The figure shows three views and two pictorial views of one solid part (mm, origin at its lowest corner). Answer the questions. A direction names the side the tool comes from. Give positions to 0.01 mm unless a question says otherwise; leave off trailing zeros. Order: outer loops, then holes, each group sorted by start corner. A loop starts at its lowest first (then second) coordinate and runs counter-clockwise, first axis right, second up. Notation, with made-up numbers: (48, -11) - (98, -11) arc R13 ccw to (98, 7) - close; hole circle Ø5 at (-35, 48.5). An arc over 180 degrees is marked (long way). Answer as CSV lines item,"result". Start each with the question number.
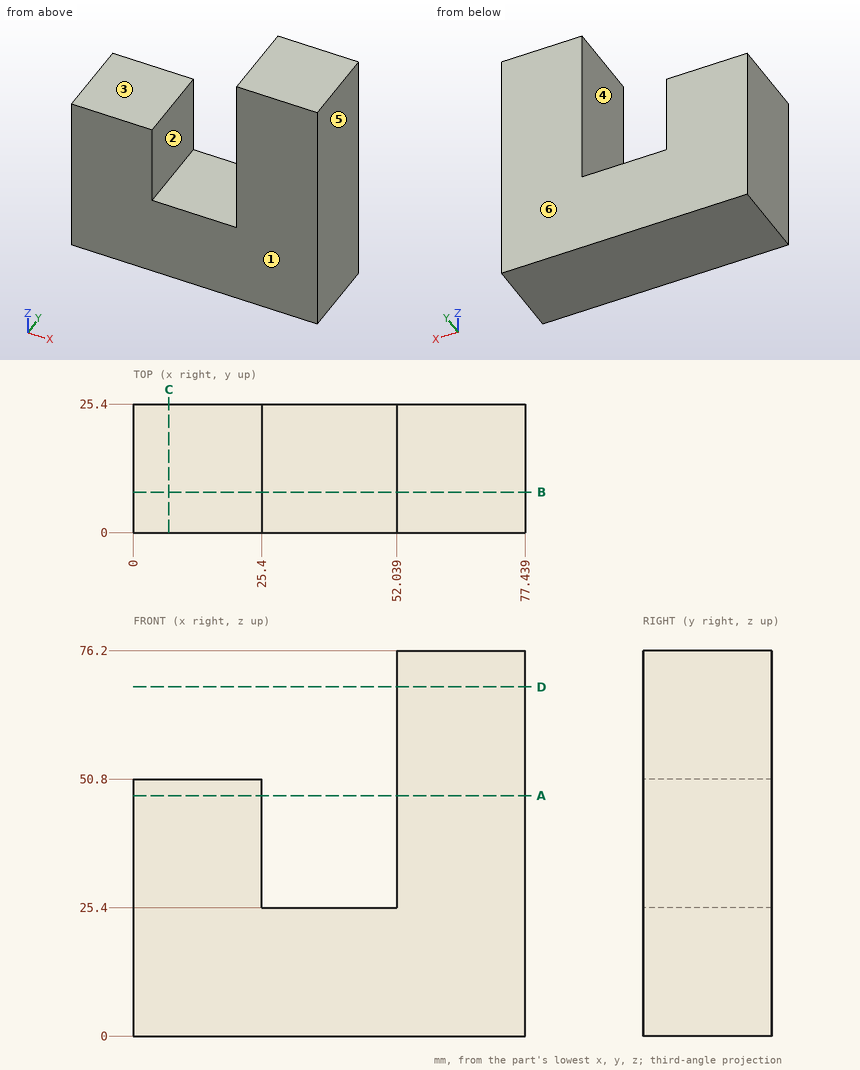
(1) Which of the six approach directions +Z, -Z, +X, -X, +Y, -Y give full straight-line access (tool end or side, diameter ignored) to the marked faces 1, 2 and 3?
(2) Section B-B, the plane y = 8 is taken. Write down the section's boundary in (x, z), and give its area (3 significant figures).
(3) Straight lines are drawn through the part: line 1 (X direction, y = 7.5, z = 48); line 2 (X direction, y = 7.25, z = 64); line 3 (Z direction, x = 42, y = 14). For each, find the intervals that lie inside material, in ascending order. Write a range as [from, to].
(4) Determine the mould class of the marked faces 4, 5 and 6 for opening direction X: released by +X, released by -X, zero draft, split by the parting line, or undercut.
(5) Flat-ended cylindrical pins translate along their axes: pin 1 Ø1.5 at (x, y) = (28, 8) entering from +Z; pin 2 Ø12.5 at (x, y) = (17, 9.5) entering from +Z; pin 3 Ø1 at (y, z) = (10, 55) entering from -X. Find the tip coordinate at first contact, or state that the pin passes through.
(6) Section C-C, the plane x = 7 is taken. Write down the section's boundary in (y, z), and give its area (3 significant figures).
(7) Section A-A, the plane z = 47.5 is taken. Write down the section's boundary in (x, y), and give its area (3 significant figures).
(8) Section D-D, the plane z = 69 is taken. Write down the section's boundary in (x, y), and give its area (3 significant figures).
Checks:
1,face 1,"+Z, -Z, +X, -X, -Y"
1,face 2,"+Z, +Y, -Y"
1,face 3,"+Z, -X, +Y, -Y"
2,outline,"(0, 0) - (77.44, 0) - (77.44, 76.2) - (52.04, 76.2) - (52.04, 25.4) - (25.4, 25.4) - (25.4, 50.8) - (0, 50.8) - close"
2,area,"3,900 mm²"
3,line 1,"x = [0, 25.4], [52.04, 77.44]"
3,line 2,"x = [52.04, 77.44]"
3,line 3,"z = [0, 25.4]"
4,face 4,"undercut"
4,face 5,"released by +X"
4,face 6,"zero draft"
5,pin 1,"stops at z = 25.4"
5,pin 2,"stops at z = 50.8"
5,pin 3,"stops at x = 52.04"
6,outline,"(0, 0) - (25.4, 0) - (25.4, 50.8) - (0, 50.8) - close"
6,area,"1,290 mm²"
7,outline,"(0, 0) - (25.4, 0) - (25.4, 25.4) - (0, 25.4) - close; (52.04, 0) - (77.44, 0) - (77.44, 25.4) - (52.04, 25.4) - close"
7,area,"1,290 mm²"
8,outline,"(52.04, 0) - (77.44, 0) - (77.44, 25.4) - (52.04, 25.4) - close"
8,area,"645 mm²"
